```python
from build123d import *

# Parameters (mm, degrees)
SKETCH1_R           = 5
BOSS_EXTRUDE1_DEPTH = 5
FILLET1_R           = 0.5
SKETCH4_R           = 1
CUT_EXTRUDE1_DEPTH  = 5


with BuildPart() as part:
    # Sketch1 → Boss-Extrude1 (new body)
    with BuildSketch(Plane.XY):
        Circle(SKETCH1_R)
    extrude(amount=BOSS_EXTRUDE1_DEPTH)

    # Sketch2 → Cut-Revolve1 (revolve, cut)
    with BuildSketch(Plane(origin=(0, 0, 0), x_dir=(0, 0, -1), z_dir=(1, 0, 0))):
        with BuildLine():
            Line((-4, 5), (-1, 5))
            ThreePointArc((-1, 5), (-2.5, 4), (-4, 5))
        make_face()
    revolve(axis=Axis((0, 0, 5.25), (0, 0, -1)), mode=Mode.SUBTRACT)

    # Fillet1
    fillet1_edges = [part.edges().sort_by_distance(p)[0] for p in [
        (-5, 0, 0),
        (-5, 0, 5),
    ]]
    fillet(fillet1_edges, radius=FILLET1_R)

    # Sketch4 → Cut-Extrude1 (cut)
    with BuildSketch(Plane.XY.offset(5)):
        Circle(SKETCH4_R)
    extrude(amount=-CUT_EXTRUDE1_DEPTH, mode=Mode.SUBTRACT)


solid = part.part
```
The listing builds one solid part. Answer for the finished solid, in the listing's coordinates (mm). Give positions to 0.01 mm unless a question says otherwise; leave off trailing zeros. Loops run counter-clockwise (first coordinate to the right, second up) from the corner with the lowest first, then second, coordinate; pieces in that order, holes last. Notation, with made-up numbers: (57.25, 73) - (75.25, 73) arc R30 cw to (75.25, 110) - close; hole circle Ø11 at (6, -12). An arc over 180 degrees is marked (long way). Answer as CSV lines item,"result". Start each with the question number.
Item 1: A cutting plane is placed at A-A on x = 0. Determine the outline of the cut face in (y, z) (3 decimals).
Item 2: A cutting plane is placed at C-C on z = 3.15. Determine the outline of the cut face in (x, y).
Item 3: Find the intervals of material crossed by line 1 (Y direction, x = 0, z = 3.1); line 2 (Z direction, x = 4.25, y = -0.5); line 3 (Y direction, x = -0.75, z = 4.1), in increasing order. Write a range as from..to.
Item 4: The mould has two halves that part along X. Classify faces 1 (the face through (1, -1, 0)), 2 (the face through (0, -1, 3)), 3 (the face through (4.619, -1.915, 4.246)): +X half, -X half, draft (parallel to the pull), parting line (faces both ways), or undercut.
Item 5: Each of these flat-tipped pins is pushed along its axis until it touches: pin 1 (3 mm diameter, centred on x = -3, z = 4, fed in from -Y); pin 2 (1.6 mm diameter, centred on x = 0, y = 0, fed in from -Z); pin 3 (2 mm diameter, centred on y = -2.5, z = 2.5, fed in from +X). Where does it stop, or does it pass through?
Item 6: A cutting plane is placed at D-D on z = 1.3. Determine the outline of the cut face in (x, y).
Found:
1,outline,"(-5, 0.5) arc R0.5 ccw to (-4.5, 0) - (-1, 0) - (-1, 5) - (-4.5, 5) arc R0.5 ccw to (-5, 4.5) - (-5, 4) arc R1.625 cw to (-5, 1) - close; (1, 0) - (4.5, 0) arc R0.5 ccw to (5, 0.5) - (5, 1) arc R1.625 cw to (5, 4) - (5, 4.5) arc R0.5 ccw to (4.5, 5) - (1, 5) - close"
2,outline,"circle Ø8.27 at (0, 0); hole circle Ø2 at (0, 0)"
3,line 1,"y = -4.11..-1, 1..4.11"
3,line 2,"z = 0..1.59, 3.41..5"
3,line 3,"y = -4.94..-0.66, 0.66..4.94"
4,face 1,"draft"
4,face 2,"undercut"
4,face 3,"parting line"
5,pin 1,"stops at y = -4.77"
5,pin 2,"passes through"
5,pin 3,"stops at x = 3.76"
6,outline,"circle Ø9.06 at (0, 0); hole circle Ø2 at (0, 0)"
